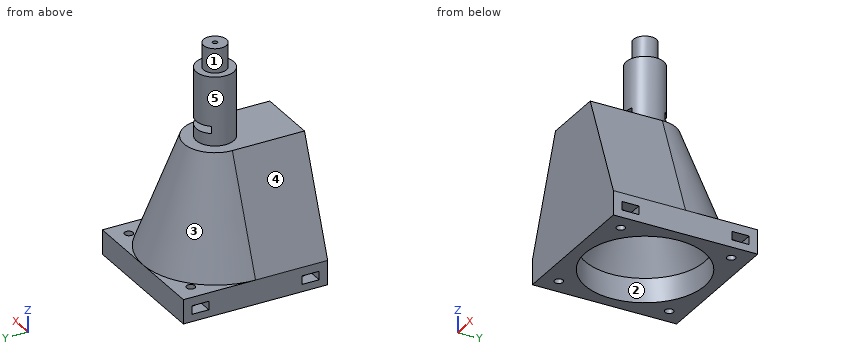
Autodesk Inventor part; units mm, degrees
ref_plane "YZ Plane" through (0, 0, 0) normal (1, 0, 0) x (0, 1, 0)
ref_plane "XZ Plane" through (0, 0, 0) normal (0, 1, 0) x (-1, 0, 0)
sketch "Sketch2" plane through (0, 0, 0) normal (0, 0, 1) x (1, 0, 0)
  line L0 (-29.75, 59.5) -> (29.75, 59.5)
  line L1 (29.75, 59.5) -> (29.75, 0)
  line L2 (29.75, 0) -> (-29.75, 0)
  line L3 (-29.75, 0) -> (-29.75, 59.5)
  point P0 (0, 0)
  point P1 (0, 0)
  dimension "d0" = 59.5
extrude "Extrusion1" add sketch "Sketch2" along normal blind 55
sketch "Sketch3" plane through (0, 0, 55) normal (0, 0, 1) x (1, 0, 0)
  circle A0 centre (0, 29.75) radius 1
  circle A1 centre (0, 29.75) radius 7.75
  line L0 (0, 0) -> (0, 59.5) construction
  line L1 (29.75, 59.5) -> (-29.75, 59.5) construction
  line L2 (29.75, 0) -> (29.75, 59.5) construction
  line L3 (29.75, 29.75) -> (-29.75, 29.75) construction
  line L4 (-29.75, 59.5) -> (-29.75, 0) construction
  line L5 (-29.75, 0) -> (29.75, 0)
  dimension "d3" = 15.5
  dimension "d5" = 2
  dimension "d47" = 22
extrude "Extrusion2" add sketch "Sketch3" along normal blind 28.3
sketch "Sketch4" plane through (0, 29.75, 83.3) normal (0, 0, 1) x (1, 0, 0)
  circle A0 centre (0, 0) radius 1
  circle A1 centre (0, 0) radius 4.75
  circle A2 centre (0, 0) radius 1
  point P0 (0, -29.75)
  dimension "d8" = 9.5
extrude "Extrusion3" add sketch "Sketch4" along normal blind 10
sketch "Sketch10" plane through (0, 0, 0) normal (0, 0, -1) x (-1, 0, 0)
  circle A0 centre (-22.75, 52.5) radius 1.75
  circle A1 centre (-22.75, 7) radius 1.75
  circle A2 centre (22.75, 52.5) radius 1.75
  circle A3 centre (22.75, 7) radius 1.75
  line L0 (-29.75, 59.5) -> (-29.75, 0)
  line L1 (29.75, 59.5) -> (-29.75, 59.5)
  line L2 (-29.75, 29.75) -> (29.75, 29.75) construction
  line L3 (29.75, 0) -> (29.75, 59.5) construction
  line L4 (0, 59.5) -> (0, 0) construction
  dimension "d29" = 7
  dimension "d30" = 7
  dimension "d33" = 3.5
extrude "Extrusion5" cut sketch "Sketch10" against normal blind 10
sketch "Sketch9" plane through (29.75, 0, 0) normal (1, 0, 0) x (0, 0, -1)
  line L0 (-6.5, 56) -> (-3, 56)
  line L1 (-3, 56) -> (-3, 49)
  line L2 (-3, 49) -> (-6.5, 49)
  line L3 (-6.5, 49) -> (-6.5, 56)
  line L4 (-6.5, 10.5) -> (-3, 10.5)
  line L5 (-3, 10.5) -> (-3, 3.5)
  line L6 (-3, 3.5) -> (-6.5, 3.5)
  line L7 (-6.5, 3.5) -> (-6.5, 10.5)
  line L8 (0, 59.5) -> (-55, 59.5)
  line L9 (-55, 0) -> (-55, 59.5) construction
  line L10 (-55, 29.75) -> (0, 29.75) construction
  line L11 (0, 0) -> (0, 59.5) construction
  line L12 (0, 54.25) -> (0, 50.75)
  line L13 (0, 52.5) -> (-10, 52.5) construction
  line L14 (-10, 54.25) -> (-10, 50.75)
  dimension "d24" = 7
  dimension "d25" = 3.5
  dimension "d26" = 3
extrude "Extrusion4" cut sketch "Sketch9" against normal blind 10
mirror "Mirror1" about plane through (0, 0, 0) normal (1, 0, 0) of "Extrusion4"
ref_plane "Work Plane1" through (0, 0, 10) normal (0, 0, 1) x (1, 0, 0)
sketch "Sketch11" plane through (0, 0, 10) normal (0, 0, 1) x (1, 0, 0)
  circle A0 centre (0, 29.75) radius 24.75
  circle A1 centre (0, 29.75) radius 1
  line L0 (-29.75, 59.5) -> (29.75, 59.5)
  point P0 (0, 0)
  dimension "d49" = 5
extrude "Extrusion6" cut sketch "Sketch11" against normal through all contours A0 | A1
loft "Loft2" cut section 1 edges at (-24.75, 29.75, 10) section 2 edges at (-1, 29.75, 55)
sketch "Sketch7" plane through (-29.75, 59.5, 0) normal (0, 1, 0) x (1, 0, 0)
  line L0 (35.75, -60) -> (23.75, -60)
  line L1 (23.75, -60) -> (23.75, -63)
  line L2 (23.75, -63) -> (35.75, -63)
  line L3 (35.75, -63) -> (35.75, -60)
  line L4 (29.75, -60) -> (29.75, -63) construction
  line L5 (26.5, -55) -> (28.5, -55) construction
  line L6 (29.75, -55) -> (29.75, -83.3) construction
  line L7 (59.5, -55) -> (0, -55) construction
  line L8 (22, -83.3) -> (37.5, -83.3)
  point P0 (29.75, 0)
  dimension "d16" = 3
  dimension "d17" = 12
  dimension "d18" = 5
extrude "Extrusion7" cut sketch "Sketch7" against normal blind 32
sketch "Sketch12" plane through (-29.75, 27.5, 0) normal (0, 1, 0) x (1, 0, 0)
  line L0 (32.75, -60) -> (26.75, -60)
  line L1 (26.75, -60) -> (26.75, -63)
  line L2 (26.75, -63) -> (32.75, -63)
  line L3 (32.75, -63) -> (32.75, -60)
  line L4 (35.75, -60) -> (35.75, -63)
  line L5 (35.75, -63) -> (23.75, -63)
  line L6 (28.75, -60) -> (30.75, -60) construction
  line L7 (29.75, -60) -> (29.75, -63) construction
  line L8 (30.75, -63) -> (28.75, -63) construction
  point P0 (29.75, 0)
  point P1 (22.3338, -63)
  dimension "d44" = 6
extrude "Extrusion8" cut sketch "Sketch12" against normal through all
sketch "Sketch14" plane through (0, 0, 0) normal (1, 0, 0) x (0, 1, 0)
  line L0 (59.5, 10) -> (42.5, 55)
  line L1 (42.5, 55) -> (79.5, 55)
  line L2 (79.5, 10) -> (79.5, 55)
  line L3 (59.5, 55) -> (0, 55)
  line L4 (37.5, 55) -> (37.5, 83.3)
  line L5 (59.5, 0) -> (59.5, 55)
  line L6 (5, 10) -> (54.5, 10)
  line L7 (79.5, 10) -> (59.5, 10)
  line L8 (59.5, 0) -> (59.5, 55)
  line L9 (54.25, 10) -> (50.75, 10)
  line L10 (29.75, -18.66) -> (29.75, 111.96)
  point P0 (0, 0)
  point P1 (55, 37.5)
  point P2 (55, 37.5)
  dimension "d54" = 5
  dimension "d55" = 20
revolve "Revolution1" cut sketch "Sketch14" angle 180 mid plane about axis through (0, 29.75, 55) along (0, 0, 1)
sketch "Sketch15" plane through (12.75, 29.75, 55) normal (0, 1, 0) x (1, 0, 0)
  line L0 (-42.5, 0) -> (-25.5, 0)
  line L1 (-25.5, 0) -> (0, 0)
  line L2 (-42.5, 0) -> (17, 0)
  line L3 (0, 0) -> (17, 0)
  line L4 (17, 0) -> (17, 45)
  line L5 (17, 55) -> (17, 0)
  line L6 (0, 0) -> (17, 45)
  line L7 (0, 0) -> (17, 45)
  line L8 (17, 45) -> (-25.5, 0)
  line L9 (-25.5, 0) -> (-42.5, 45)
  line L10 (-42.5, 45) -> (-25.5, 0)
  line L11 (-42.5, 0) -> (-42.5, 45)
  line L12 (-42.5, 55) -> (-42.5, 0)
  point P0 (-12.75, 55)
extrude "Extrusion10" cut sketch "Sketch15" against normal through all contours L11 L9 L0 | L6 L4 L2
properties part number "Power_Meter_Adapter_Part1"
Can you work these out from the model? Positions are in its coordinate system, mm. Face numbers are marked on the shaded views. A direction names the side the tool comes from. Give positions to 0.01 mm unless a question says otherwise; leave off trailing zeros. Loops run counter-clockwise (first coordinate to the right, second up) from the corner with the lowest first, then second, coordinate; pieces in that order, holes last. Notation, with made-up numbers: (-29, 29.25) - (13, 29.25) arc R13 ccw to (13, 36.25) - close; hole circle Ø1 at (68, 27). An arc over 180 degrees is marked (long way). Return JSON: item names as keys, results as strings.
1. For the marked faces 4 and 5, which set-ups out of +Z, -Z, +X, -X, +Y, -Y let a thin tool reach every point of the face, with its end or its side?
Output values:
{"face 4": "+Z, -X, +Y, -Y", "face 5": "+Z"}
2. We'd pull the mould along Y, two halves only. Please class the marked faces 1, 2 and 3: +Y half, -Y half, draft (parallel to the pull), parting line (faces both ways), or undercut.
Output values:
{"face 1": "parting line", "face 2": "undercut", "face 3": "+Y half"}
3. I'm going to push flat-ended pins straight in: pin 1 Ø1 at (x, z) = (23.5, 5) entering from -Y; pin 2 Ø8 at (x, y) = (14.5, 39.5) entering from -Z; pin 3 Ø10 at (x, y) = (-8, 36) entering from -Z; pin 4 Ø12 at (x, y) = (8.5, 40.5) entering from -Z. Where does each tip first touch, or does it pass through?
Output values:
{"pin 1": "stops at y = 0", "pin 2": "stops at z = 16.21", "pin 3": "stops at z = 28.19", "pin 4": "stops at z = 19.56"}
4. I want a section at B-B on y = 7. Give the number of separate pieces and of enclosed holes in the cut face, and give its area (3 significant figures).
Output values:
{"separate pieces": "3", "enclosed holes": "0", "area": "2,150 mm²"}
5. If I drill on line 1 (Y direction, x = 0, z = 7.5); line 2 (Y direction, x = 22.75, z = 1.1); line 3 (Y direction, x = -22, z = 1), over which ranges is the centre line in solid material (lowest first)?
Output values:
{"line 1": "y = 0 to 5, 54.5 to 59.5", "line 2": "y = 0 to 5.25, 8.75 to 20, 39.5 to 50.75, 54.25 to 59.5", "line 3": "y = 0 to 5.42, 8.58 to 18.41, 41.09 to 50.92, 54.08 to 59.5"}
6. I want a section at C-C on z = 27. Please give me the cut outline in (x, y).
Output values:
{"outline": "(-23.33, 0) - (23.33, 0) - (23.33, 29.75) arc R23.33 ccw to (-23.33, 29.75) - close; hole circle Ø31.56 at (0, 29.75)"}
7. I want a section at A-A on z = 8. Please give me the cut outline in (x, y), and give its area (3 significant figures).
Output values:
{"outline": "(-29.75, 0) - (29.75, 0) - (29.75, 59.5) - (-29.75, 59.5) - close; hole circle Ø49.5 at (0, 29.75); hole circle Ø3.5 at (-22.75, 7); hole circle Ø3.5 at (-22.75, 52.5); hole circle Ø3.5 at (22.75, 7); hole circle Ø3.5 at (22.75, 52.5)", "area": "1,580 mm²"}
